Could you check a few things on this model? Use its own coordinates, in mm. Face numbers are marked on the shaded views. Give positions to 0.01 mm unless a question says otherwise; leave off trailing zeros. Loops run counter-clockwise (first coordinate to the right, second up) from the corner with the lowest first, then second, coordinate; pieces in that order, holes last. Notation, with made-up numbers: M 57.25,7 L 68.25,7 A15 cw 68.25,35 Z; hole C 55.5,-39 d3. An arc over 180 degrees is marked long. Use a Markdown table: item, result. Add a question column.
1) Suppose I cut it at C-C on z = -18. List the corners of the cut face in (x, y) for me, and give its area (3 significant figures).
2) Suppose I cut it at A-A on y = 5. Count the separate pieces of the cut face and the enclosed holes in it, and give its area (3 significant figures).
3) If I drill on line 1 along Z through (x, y) = (-32.5, 6); line 2 along X through (y, z) = (5.75, 12.5); line 3 along X through (y, z) = (5.5, 22), over which ranges is the centre line in solid material (lowest first)? Write a range as [from, to].
4) We'd pull the mould along Z, two halves only. Please class the marked faces 1, 2, 3 and 4: +Z half, -Z half, draft (parallel to the pull), parting line (faces both ways), or undercut.
5) Will these pins go through, and if not, where does the flat tip stop? pin 1 Ø5.5 at (x, z) = (-10.06, -27.61) entering from +Y; pin 2 Ø8 at (x, z) = (2.5, 21) entering from +Y; pin 3 Ø5.5 at (x, z) = (-68.06, -27.61) entering from -Y.
6) Suppose I cut it at B-B on x = -25.5. List the corners of the cut face in (y, z) for me.
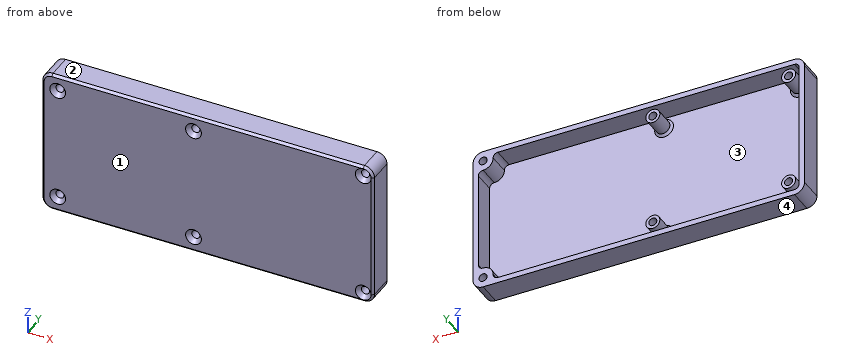
```python
from build123d import *

# Parameters (mm, degrees)
SKETCH3_W                                         = 141.6
SKETCH3_H                                         = 62.6
SKETCH3_W_2                                       = 137
SKETCH3_H_2                                       = 58
BOSS_EXTRUDE1_DEPTH                               = 11.3
SKETCH5_W                                         = 137
SKETCH5_H                                         = 58
BOSS_EXTRUDE2_DEPTH                               = 2
SKETCH6_R                                         = 3
BOSS_EXTRUDE3_DEPTH                               = 9.3
FILLET6_R                                         = 2
FILLET8_R                                         = 2
CHAMFER1_SIZE                                     = 1
SKETCH24_R                                        = 4.3
BOSS_EXTRUDE7_DEPTH                               = 9.3
FILLET21_R                                        = 2
FILLET22_R                                        = 2
FILLET20_R                                        = 4.3
CSK_FOR_4_FLAT_HEAD_SOCKET_CAP_SCREW1_D           = 3.4544
CSK_FOR_4_FLAT_HEAD_SOCKET_CAP_SCREW1_DEPTH       = 14
CSK_FOR_4_FLAT_HEAD_SOCKET_CAP_SCREW1_CSINK_D     = 6.723761
CSK_FOR_4_FLAT_HEAD_SOCKET_CAP_SCREW1_CSINK_ANGLE = 82
CSK_FOR_4_FLAT_HEAD_SOCKET_CAP_SCREW1_TIP         = 1.037806461
CHAMFER7_SIZE                                     = 1


# Some blends are built 0.0001 mm under size
with BuildPart() as part:
    # Sketch3 → Boss-Extrude1 (new body)
    with BuildSketch(Plane(origin=(0, 0, 0), x_dir=(1, 0, 0), z_dir=(0, 1, 0))):
        with Locations((-4.061766162, 3.105993834)):
            Rectangle(SKETCH3_W, SKETCH3_H)
        with Locations((-4.061766162, 3.105993834)):
            Rectangle(SKETCH3_W_2, SKETCH3_H_2, mode=Mode.SUBTRACT)
    extrude(amount=BOSS_EXTRUDE1_DEPTH)

    # Sketch5 → Boss-Extrude2 (add)
    with BuildSketch(Plane(origin=(0, 0, 0), x_dir=(1, 0, 0), z_dir=(0, 1, 0))):
        with Locations((-4.061766162, 3.105993834)):
            Rectangle(SKETCH5_W, SKETCH5_H)
    extrude(amount=BOSS_EXTRUDE2_DEPTH)

    # Sketch6 → Boss-Extrude3 (add)
    with BuildSketch(Plane(origin=(0, 2, 0), x_dir=(1, 0, 0), z_dir=(0, 1, 0))):
        with Locations(Location((-68.061766162, 27.605993834, 0), (0, 0, 270))):
            Circle(SKETCH6_R)
        with Locations(Location((-68.061766162, -21.394006166, 0), (0, 0, 270))):
            Circle(SKETCH6_R)
        with Locations(Location((-10.061766162, -21.394006166, 0), (0, 0, 270))):
            Circle(SKETCH6_R)
        with Locations(Location((-10.061766162, 27.605993834, 0), (0, 0, 270))):
            Circle(SKETCH6_R)
    extrude(amount=BOSS_EXTRUDE3_DEPTH)

    # Fillet6
    fillet6_edges = [part.edges().sort_by_distance(p)[0] for p in [
        (64.438233838, 6.65, -32.105993834),
    ]]
    fillet(fillet6_edges, radius=FILLET6_R)

    # Fillet8
    fillet8_edges = [part.edges().sort_by_distance(p)[0] for p in [
        (-72.561766162, 6.65, -32.105993834),
        (-72.561766162, 6.65, 25.894006166),
    ]]
    fillet(fillet8_edges, radius=FILLET8_R)

    # Chamfer1
    chamfer1_edges = [part.edges().sort_by_distance(p)[0] for p in [
        (-68.061766162, 2, -30.605993834),
        (-68.061766162, 2, 18.394006166),
        (-10.061766162, 2, 18.394006166),
        (-10.061766162, 2, -30.605993834),
    ]]
    chamfer(chamfer1_edges, length=CHAMFER1_SIZE)

    # Sketch24 → Boss-Extrude7 (add)
    with BuildSketch(Plane(origin=(0, 2, 0), x_dir=(1, 0, 0), z_dir=(0, 1, 0))):
        with Locations((62.438233838, -23.894006166)):
            Circle(SKETCH24_R)
        with Locations((62.438233838, 30.01834388)):
            Circle(SKETCH24_R)
    extrude(amount=BOSS_EXTRUDE7_DEPTH)

    # Fillet21
    fillet21_edges = [part.edges().sort_by_distance(p)[0] for p in [
        (58.631660576, 6.65, 25.894006166),
    ]]
    fillet(fillet21_edges, radius=FILLET21_R)

    # Fillet22
    fillet22_edges = [part.edges().sort_by_distance(p)[0] for p in [
        (64.438233838, 6.65, -26.211770618),
        (58.679016144, 6.65, -32.105993834),
        (64.438233838, 6.65, 20.087432904),
    ]]
    fillet(fillet22_edges, radius=FILLET22_R)

    # Fillet20
    fillet20_edges = [part.edges().sort_by_distance(p)[0] for p in [
        (-74.861766162, 5.65, -34.405993834),
        (66.738233838, 5.65, -34.405993834),
        (66.738233838, 5.65, 28.194006166),
        (-74.861766162, 5.65, 28.194006166),
    ]]
    fillet(fillet20_edges, radius=FILLET20_R - 0.0001)  # a hair under: the kernel refuses the full size

    # CSK for #4 Flat Head Socket Cap Screw1
    with Locations(Plane(origin=(0, 0, 0), x_dir=(-1, 0, 0), z_dir=(0, -1, 0))):
        with Locations((68.061766162, 27.605993834), (68.061766162, -21.394006166), (-62.438233838, 30.105993834), (-62.438233838, -23.894006166), (10.061766162, -21.394006166), (10.061766162, 27.605993834)):
            CounterSinkHole(CSK_FOR_4_FLAT_HEAD_SOCKET_CAP_SCREW1_D / 2, CSK_FOR_4_FLAT_HEAD_SOCKET_CAP_SCREW1_CSINK_D / 2, depth=CSK_FOR_4_FLAT_HEAD_SOCKET_CAP_SCREW1_DEPTH, counter_sink_angle=CSK_FOR_4_FLAT_HEAD_SOCKET_CAP_SCREW1_CSINK_ANGLE)
            with Locations((0, 0, -(CSK_FOR_4_FLAT_HEAD_SOCKET_CAP_SCREW1_DEPTH + CSK_FOR_4_FLAT_HEAD_SOCKET_CAP_SCREW1_TIP / 2))):  # 118° drill point
                Cone(0, CSK_FOR_4_FLAT_HEAD_SOCKET_CAP_SCREW1_D / 2, CSK_FOR_4_FLAT_HEAD_SOCKET_CAP_SCREW1_TIP, mode=Mode.SUBTRACT)

    # Chamfer7
    # the kernel refuses this chamfer: 1 mm, written as the material it takes off along each edge
    with BuildSketch(Plane(origin=(62.438333838, 0, -34.405993834), x_dir=(0, -0.027495876610586292, 0.9996219169112968), z_dir=(-1, 0, 0)), Plane(origin=(-70.561866162, 0, 28.194006166), x_dir=(0, -0.02749587661058639, -0.9996219169112968), z_dir=(1, 0, 0))) as chamfer7_piece_1:
        Polygon((CHAMFER7_SIZE * 0.999621916911, CHAMFER7_SIZE * 0.0274958766106), (-CHAMFER7_SIZE * 0.0274958766106, CHAMFER7_SIZE * 0.999621916911), (0, 0), align=None)
    extrude(amount=133.0002, mode=Mode.SUBTRACT)
    with BuildSketch(Plane(origin=(-74.861766162, 0, -30.106093834), x_dir=(0.9996219169112968, -0.027495876610586483, 0), z_dir=(0, 0, 1)), Plane(origin=(66.738233838, 0, 23.894106166), x_dir=(-0.9996219169112968, -0.027495876610586483, 0), z_dir=(0, 0, -1))) as chamfer7_piece_2:
        Polygon((CHAMFER7_SIZE * 0.999621916911, CHAMFER7_SIZE * 0.0274958766106), (-CHAMFER7_SIZE * 0.0274958766106, CHAMFER7_SIZE * 0.999621916911), (0, 0), align=None)
    extrude(amount=54.0002, mode=Mode.SUBTRACT)
    with BuildSketch(Plane(origin=(62.438333838, 0, 23.894106166), x_dir=(0, 0, 1), z_dir=(-1, 0, 0))) as chamfer7_piece_3:
        Polygon((4.2999 - CHAMFER7_SIZE, 0), (4.2999, CHAMFER7_SIZE), (4.2999, 0), align=None)
    revolve(axis=Axis((62.438333838, 0, 23.894106166), (0, 1, 0)), revolution_arc=90, mode=Mode.SUBTRACT)
    with BuildSketch(Plane(origin=(-70.561866162, 0, 23.894106166), x_dir=(0, 0, 1), z_dir=(1, 0, 0))) as chamfer7_piece_4:
        Polygon((4.2999 - CHAMFER7_SIZE, 0), (4.2999, -CHAMFER7_SIZE), (4.2999, 0), align=None)
    revolve(axis=Axis((-70.561866162, 0, 23.894106166), (0, -1, 0)), revolution_arc=90, mode=Mode.SUBTRACT)
    with BuildSketch(Plane(origin=(-70.561866162, 0, -30.106093834), x_dir=(0, 0, -1), z_dir=(1, 0, 0))) as chamfer7_piece_5:
        Polygon((4.2999 - CHAMFER7_SIZE, 0), (4.2999, CHAMFER7_SIZE), (4.2999, 0), align=None)
    revolve(axis=Axis((-70.561866162, 0, -30.106093834), (0, 1, 0)), revolution_arc=90, mode=Mode.SUBTRACT)
    with BuildSketch(Plane(origin=(62.438333838, 0, -30.106093834), x_dir=(1, 0, 0), z_dir=(0, 0, 1))) as chamfer7_piece_6:
        Polygon((4.2999 - CHAMFER7_SIZE, 0), (4.2999, CHAMFER7_SIZE), (4.2999, 0), align=None)
    revolve(axis=Axis((62.438333838, 0, -30.106093834), (0, 1, 0)), revolution_arc=90, mode=Mode.SUBTRACT)


solid = part.part
```
Answer block:
| question | item | result |
|---|---|---|
| 1 | outline | M -74.86,1 L -73.86,0 L 65.74,0 L 66.74,1 L 66.74,11.3 L 64.44,11.3 L 64.44,2 L -72.56,2 L -72.56,11.3 L -74.86,11.3 Z |
| 1 | area | 325 mm^2 |
| 2 | separate pieces | 5 |
| 2 | enclosed holes | 7 |
| 2 | area | 1,040 mm^2 |
| 3 | line 1 | z = [-34.41, -32.11], [25.89, 28.19] |
| 3 | line 2 | x = [-74.86, -72.56], [64.44, 66.74] |
| 3 | line 3 | x = [-74.86, -72.56], [-71, -69.68], [-66.44, -65.12], [-13, -11.68], [-8.44, -7.12], [58.58, 66.74] |
| 4 | face 1 | draft |
| 4 | face 2 | +Z half |
| 4 | face 3 | undercut |
| 4 | face 4 | -Z half |
| 5 | pin 1 | stops at y = 11.3 |
| 5 | pin 2 | stops at y = 2 |
| 5 | pin 3 | stops at y = 0.7 |
| 6 | outline | M 0,-33.41 L 1,-34.41 L 11.3,-34.41 L 11.3,-32.11 L 2,-32.11 L 2,25.89 L 11.3,25.89 L 11.3,28.19 L 1,28.19 L 0,27.19 Z |
